Source: CAD feature listing. Evaluate the final solid. Frame: model axes, mm. Face numbers are marked on the shaded views. Round coordinates to 2 decimals unless told otherwise and drop trailing zeros. Order: outer loops, then holes, each group sorted by start corner. A loop starts at its lowest first (then second) coordinate and runs counter-clockwise, first axis right, second up. Notation, with made-up numbers: (86, -7) - (109, -7) arc R21 cw to (109, 29) - close; hole circle Ø4 at (87.25, 77). An arc over 180 degrees is marked (long way). Return JSON: item names as keys, results as strings. Group by question number.
1) Contact query for flat-ended pins moving along their axis: P1, Ø1.5, axis at y = 7.5, z = 5, coming from the +X side; P2, Ø0.6, axis at x = 32.5, z = 5, coming from the -Y side; P3, Ø6, axis at y = 1, z = 21, coming from the -X side. Output: stop coordinate, or through.
2) Section A-A, the plane y = 0. Return loops of the section in (x, z), plus the area to 3 significant figures.
3) Section D-D, the plane x = 25. Return loops of the section in (y, z), plus the area to 3 significant figures.
4) Section C-C, the plane x = -21. Return loops of the section in (y, z), plus the area to 3 significant figures.
5) Ray query, line 1 (Y direction, x = 0, z = 30.5); line 2 (Z direction, x = -36.5, y = -3.5); line 3 (Y direction, x = 9.5, z = 18.5). Return the intervals inside material, ascending. Write a range as from..to.
6) Mould query, pull axis Y, two halves, no side actions, for the marked faces 1 and 2. Classes: pulls with the +Y half, pulls with the -Y half, needs draft (parallel to the pull), parting line crosses it, or undercut.
7) Section B-B, the plane z = 39. Return loops of the section in (x, y).
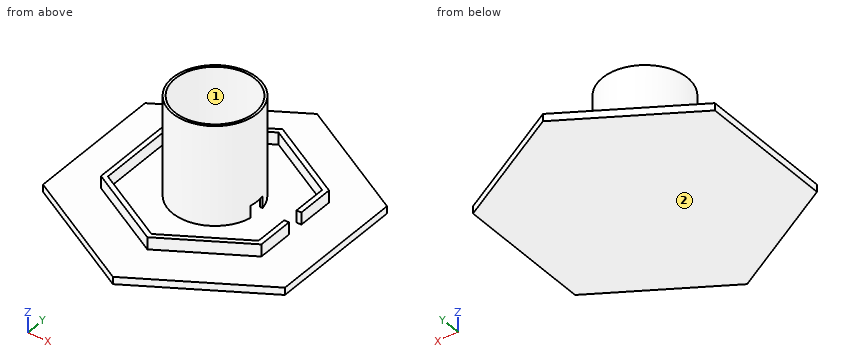
```python
from build123d import *

# Parameters (mm, degrees)
F1_DEPTH = 3
F3_DEPTH = 5
F5_DEPTH = 5
F6_R     = 17.5
F6_R_2   = 16.5
F7_DEPTH = 41
F8_W     = 3.5
F8_H     = 4
F9_DEPTH = 25


with BuildPart() as f1:
    # F0 (on Top) → F1 (new body)
    with BuildSketch(Plane.XY):
        Polygon((49.999933, 28.867475), (0, 57.73495), (-49.999933, 28.867475), (-49.999933, -28.867475), (0, -57.73495), (49.999933, -28.867475), align=None)
    extrude(amount=F1_DEPTH)

    # F2 (on face) → F3 (join)
    with BuildSketch(Plane.XY.offset(3)):
        Polygon((33.143658, 19.1355), (0, 38.271), (-33.143658, 19.1355), (-33.143658, -19.1355), (0, -38.271), (33.143658, -19.1355), align=None)
    extrude(amount=F3_DEPTH)

    # F4 (on face) → F5 (cut)
    with BuildSketch(Plane.XY.offset(8)):
        Polygon((31.143884, 17.98093), (0, 35.96186), (-31.143884, 17.98093), (-31.143884, -17.98093), (0, -35.96186), (31.143884, -17.98093), align=None)
    extrude(amount=-F5_DEPTH, mode=Mode.SUBTRACT)

    # F6 (on face) → F7 (join)
    with BuildSketch(Plane.XY.offset(3)):
        Circle(F6_R)
        Circle(F6_R_2, mode=Mode.SUBTRACT)
    extrude(amount=F7_DEPTH)

    # F8 (on face) → F9 (cut)
    with BuildSketch(Plane.YZ.offset(33.143658)):
        with Locations((-1.75, 5)):
            Rectangle(F8_W, F8_H)
        with Locations((1.75, 5)):
            Rectangle(F8_W, F8_H)
        Polygon((-3.5, 7), (0, 7), (3.5, 7), (3.5, 8), (-3.5, 8), align=None)
    extrude(amount=-F9_DEPTH, mode=Mode.SUBTRACT)


solid = f1.part
```
Geometry check:
{
 "1": {"P1": "x = 33.14", "P2": "y = -19.68", "P3": "x = -17.5"},
 "2": {"outline": "(-50, 0) - (50, 0) - (50, 3) - (-16.5, 3) - (-16.5, 44) - (-17.5, 44) - (-17.5, 3) - (-31.14, 3) - (-31.14, 8) - (-33.14, 8) - (-33.14, 3) - (-50, 3) - close; (16.5, 8) - (17.5, 8) - (17.5, 44) - (16.5, 44) - close", "area": "387 mm2"},
 "3": {"outline": "(-43.3, 0) - (43.3, 0) - (43.3, 3) - (23.84, 3) - (23.84, 8) - (21.53, 8) - (21.53, 3) - (-21.53, 3) - (-21.53, 8) - (-23.84, 8) - (-23.84, 3) - (-43.3, 3) - close", "area": "283 mm2"},
 "4": {"outline": "(-45.61, 0) - (45.61, 0) - (45.61, 3) - (26.15, 3) - (26.15, 8) - (23.84, 8) - (23.84, 3) - (-23.84, 3) - (-23.84, 8) - (-26.15, 8) - (-26.15, 3) - (-45.61, 3) - close", "area": "297 mm2"},
 "5": {"line 1": "-17.5..-16.5, 16.5..17.5", "line 2": "0..3", "line 3": "-14.7..-13.49, 13.49..14.7"},
 "6": {"face 1": "undercut", "face 2": "needs draft"},
 "7": {"outline": "circle Ø35 at (0, 0); hole circle Ø33 at (0, 0)"}
}
